from build123d import *

# Parameters (mm, degrees)
SKETCH1_W           = 6.5
SKETCH1_H           = 20.7
BOSS_EXTRUDE1_DEPTH = 10.1
FILLET1_SIZE        = 4
FILLET1_SIZE_2      = 6.5
FILLET2_SIZE        = 3.5
FILLET2_SIZE_2      = 6.5
SKETCH4_R           = 1.75
BOSS_EXTRUDE3_DEPTH = 2.7
FILLET4_R           = 0.15
SKETCH2_W           = 20.7
SKETCH2_H           = 10.1
CUT_EXTRUDE1_DEPTH  = 12.8
SKETCH5_R           = 3.5
CUT_EXTRUDE2_DEPTH  = 13.3
SKETCH6_R           = 3.1
SKETCH6_R_2         = 2.8
BOSS_EXTRUDE4_DEPTH = 12


with BuildPart() as part:
    # Sketch1 → Boss-Extrude1 (new body)
    with BuildSketch(Plane(origin=(0, 0, 0), x_dir=(1, 0, 0), z_dir=(0, 1, 0))):
        Polygon((-2.6, 10.35), (-7.1, 10.35), (-7.1, -10.35), (-2.6, -10.35), (-2.6, -9.975), (-3.1, -9.975), (-3.1, -9.225), (-1.1, -9.225), (-1.1, -9.975), (-1.6, -9.975), (-1.6, -10.35), (13.6, -10.35), (13.6, 10.35), (-1.6, 10.35), (-1.6, 9.975), (-1.1, 9.975), (-1.1, 9.225), (-3.1, 9.225), (-3.1, 9.975), (-2.6, 9.975), align=None)
        with Locations((-10.35, 0)):
            Rectangle(SKETCH1_W, SKETCH1_H)
    extrude(amount=BOSS_EXTRUDE1_DEPTH)

    # Fillet1
    # a fillet whose section is not a circle: 6.5, 4 mm, written as the material it takes off along each edge
    with BuildSketch(Plane(origin=(-13.6, 10.1, -26.6), x_dir=(0, -1, 0), z_dir=(0, 0, 1))) as fillet1_piece_1:
        with BuildLine():
            Bezier((FILLET1_SIZE, 0), (0, 0), (0, FILLET1_SIZE_2), weights=[1, 0.707106781, 1])
            Line((0, FILLET1_SIZE_2), (0, 0))
            Line((0, 0), (FILLET1_SIZE, 0))
        make_face()
    extrude(amount=53.2, mode=Mode.SUBTRACT)

    # Fillet2
    # a fillet whose section is not a circle: 6.5, 3.5 mm, written as the material it takes off along each edge
    with BuildSketch(Plane(origin=(-13.6, -16.25, 10.35), x_dir=(0, 0, -1), z_dir=(0, 1, 0))) as fillet2_piece_1:
        with BuildLine():
            Bezier((FILLET2_SIZE, 0), (0, 0), (0, -FILLET2_SIZE_2), weights=[1, 0.707106781, 1])
            Line((0, -FILLET2_SIZE_2), (0, 0))
            Line((0, 0), (FILLET2_SIZE, 0))
        make_face()
    extrude(amount=38.6, mode=Mode.SUBTRACT)
    with BuildSketch(Plane(origin=(-13.6, -16.25, -10.35), x_dir=(1, 0, 0), z_dir=(0, 1, 0))) as fillet2_piece_2:
        with BuildLine():
            Bezier((FILLET2_SIZE_2, 0), (0, 0), (0, -FILLET2_SIZE), weights=[1, 0.707106781, 1])
            Line((0, -FILLET2_SIZE), (0, 0))
            Line((0, 0), (FILLET2_SIZE_2, 0))
        make_face()
    extrude(amount=38.6, mode=Mode.SUBTRACT)

    # Sketch4 → Boss-Extrude3 (add)
    with BuildSketch(Plane.XZ):
        with Locations(Location((-11.1, -5.65, 0), (0, 0, 90))):
            Circle(SKETCH4_R)
        with Locations(Location((-11.1, 5.65, 0), (0, 0, 90))):
            Circle(SKETCH4_R)
    extrude(amount=BOSS_EXTRUDE3_DEPTH)

    # Fillet4
    fillet4_edges = [part.edges().sort_by_distance(p)[0] for p in [
        (-11.1, -2.7, -7.4),
        (-11.1, -2.7, 3.9),
    ]]
    fillet(fillet4_edges, radius=FILLET4_R)

    # Sketch2 → Cut-Extrude1 (cut)
    with BuildSketch(Plane(origin=(13.6, 0, 0), x_dir=(0, 0, -1), z_dir=(1, 0, 0))):
        with Locations((0, 5.05)):
            Rectangle(SKETCH2_W, SKETCH2_H)
        Polygon((-9.65, 7.4), (-9.65, 2.7), (-6.75, 0.6), (6.85, 0.6), (9.75, 0.6), (9.75, 9.5), (6.85, 9.5), (-6.75, 9.5), align=None, mode=Mode.SUBTRACT)
    extrude(amount=-CUT_EXTRUDE1_DEPTH, mode=Mode.SUBTRACT)

    # Sketch5 → Cut-Extrude2 (cut)
    with BuildSketch(Plane(origin=(13.6, 0, 0), x_dir=(0, 0, -1), z_dir=(1, 0, 0))):
        with Locations((-5.45, 5.05)):
            Circle(SKETCH5_R)
        with Locations((5.45, 5.05)):
            Circle(SKETCH5_R)
    extrude(amount=-CUT_EXTRUDE2_DEPTH, mode=Mode.SUBTRACT)

    # Sketch6 → Boss-Extrude4 (add)
    # profile 1 of 2: a face of its own
    with BuildSketch(Plane(origin=(0.3, 0, 0), x_dir=(0, 0, -1), z_dir=(1, 0, 0))):
        with Locations((-5.45, 5.05)):
            Circle(SKETCH6_R)
        with Locations((-5.45, 5.05)):
            Circle(SKETCH6_R_2, mode=Mode.SUBTRACT)
    # profile 2 of 2: a face of its own
    with BuildSketch(Plane(origin=(0.3, 0, 0), x_dir=(0, 0, -1), z_dir=(1, 0, 0))):
        with Locations((5.45, 5.05)):
            Circle(SKETCH6_R)
        with Locations((5.45, 5.05)):
            Circle(SKETCH6_R_2, mode=Mode.SUBTRACT)
    extrude(amount=BOSS_EXTRUDE4_DEPTH)


solid = part.part
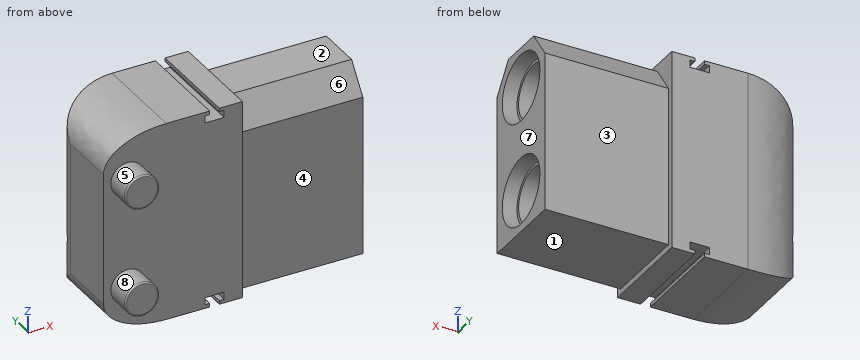
Geometry check sheet. Reference: the model listing, model coordinates, mm. Face numbers are marked on the shaded views. A direction names the side the tool comes from. Give positions to 0.01 mm unless a question says otherwise; leave off trailing zeros. Loops run counter-clockwise (first coordinate to the right, second up) from the corner with the lowest first, then second, coordinate; pieces in that order, holes last. Notation, with made-up numbers: (72, -28) -> (89, -28) arc R10 cw to (89, -16) -> close; hole circle Ø10 at (-23, 4). An arc over 180 degrees is marked (long way). Answer in a Markdown table with one row per item. Add a question column.
1) Material ranges on probe 1 along Y at (x, z) = (5.75, -5.45); probe 2 along Y at (x, z) = (7, -7.5); probe 3 along Y at (x, z) = (10, -1.5), recorded low to high. Write a range as from..to.
2) Gauge pin test, flat ends, axial feed: P1, Ø10, axis at x = -2.5, z = 1.5, coming from the -Y side; P2, Ø3, axis at y = 5, z = -6.5, coming from the +X side; P3, Ø1.5, axis at x = 2, z = 1.5, coming from the +Y side. Record the tip position at first contact, or that the pin passes through.
3) Set-up check for the marked faces 1, 2, 3, 4 and 5: record each of +Z, -Z, +X, -X, +Y, -Y from which the full face is reachable in a straight line by a thin tool's end or side.
4) Cross-section at A-A on x = 11.5. Record the boundary of the cut face in (y, z), and give its area (3 significant figures).
5) Draft check along Z on the marked faces 6, 7 and 8. Enter one of: pulls with the +Z half, pulls with the -Z half, needs draft (parallel to the pull), parting line crosses it, or undercut.
Outcome:
| question | item | result |
|---|---|---|
| 1 | probe 1 | y = 0.6..1.55, 1.95..2.25, 7.85..8.15, 8.55..9.5 |
| 1 | probe 2 | y = 0.6..2.21, 2.72..3.14, 6.96..7.38, 7.89..9.5 |
| 1 | probe 3 | y = 0.6..9.5 |
| 2 | P1 | stops at y = 0 |
| 2 | P2 | stops at x = 0.3 |
| 2 | P3 | stops at y = 9.5 |
| 3 | face 1 | -Z, +X, +Y, -Y |
| 3 | face 2 | +Z, +X, +Y, -Y |
| 3 | face 3 | +Z, -Z, +X, +Y |
| 3 | face 4 | +Z, -Z, +X, -Y |
| 3 | face 5 | -Y |
| 4 | outline | (0.6, -9.75) -> (9.5, -9.75) -> (9.5, 6.75) -> (7.4, 9.65) -> (2.7, 9.65) -> (0.6, 6.75) -> close; circle Ø6.2 at (5.05, -5.45); circle Ø6.2 at (5.05, 5.45); hole circle Ø7 at (5.05, -5.45); hole circle Ø7 at (5.05, 5.45); hole circle Ø5.6 at (5.05, -5.45); hole circle Ø5.6 at (5.05, 5.45) |
| 4 | area | 101 mm^2 |
| 5 | face 6 | pulls with the +Z half |
| 5 | face 7 | needs draft |
| 5 | face 8 | undercut |
